from build123d import *

# Parameters (mm, degrees)
SKETCH1_W           = 62
SKETCH1_H           = 42
SKETCH1_W_2         = 41
SKETCH1_H_2         = 21
BOSS_EXTRUDE1_DEPTH = 42
SKETCH2_W           = 4
SKETCH2_H           = 25
BOSS_EXTRUDE2_DEPTH = 4.5
SKETCH2_2_W         = 4
SKETCH2_2_H         = 25
BOSS_EXTRUDE3_DEPTH = 45.55
SKETCH3_W           = 4
SKETCH3_H           = 25
BOSS_EXTRUDE6_DEPTH = 2
SKETCH3_8_W         = 4
SKETCH3_8_H         = 25
BOSS_EXTRUDE7_DEPTH = 53
CUT_EXTRUDE1_DEPTH  = 51
SKETCH_1_W          = 8.5
SKETCH_1_H          = 5.5
CUT_EXTRUDE_1_DEPTH = 40
CUT_EXTRUDE_3_DEPTH = 42
EXTRUDE_1_DEPTH     = 13.5
CUT_EXTRUDE_4_DEPTH = 11.5


with BuildPart() as part:
    # Sketch1 → Boss-Extrude1 (new body)
    with BuildSketch(Plane.XY):
        with Locations((1.904162196, -4.136072895)):
            Rectangle(SKETCH1_W, SKETCH1_H)
        with Locations((1.904162196, -4.136072895)):
            Rectangle(SKETCH1_W_2, SKETCH1_H_2, mode=Mode.SUBTRACT)
    extrude(amount=BOSS_EXTRUDE1_DEPTH)

    # Sketch2 → Boss-Extrude2 (add)
    with BuildSketch(Plane.XY.offset(42)):
        with Locations((-27.095837804, -4.136072895)):
            Rectangle(SKETCH2_W, SKETCH2_H)
    extrude(amount=BOSS_EXTRUDE2_DEPTH)

    # Sketch2_2 → Boss-Extrude3 (add)
    with BuildSketch(Plane.XY.offset(42)):
        with Locations((-27.095837804, -4.136072895)):
            Rectangle(SKETCH2_2_W, SKETCH2_2_H)
    extrude(amount=-BOSS_EXTRUDE3_DEPTH)

    # Sketch3 → Boss-Extrude6 (add)
    with BuildSketch(Plane.XY.offset(46.5)):
        with BuildLine():
            Line((-60.095837804, 4.463927105), (-60.095837804, 8.363927105))
            ThreePointArc((-60.095837804, 8.363927105), (-72.595837804, -4.136072895), (-60.095837804, -16.636072895))
            Line((-60.095837804, -16.636072895), (-60.095837804, -13.176248856))
            Line((-60.095837804, -13.176248856), (-60.555926168, -13.176248856))
            ThreePointArc((-60.555926168, -13.176248856), (-62.055926168, -11.676248856), (-60.555926168, -10.176248856))
            Line((-60.555926168, -10.176248856), (-60.095837804, -10.176248856))
            Line((-60.095837804, -10.176248856), (-60.095837804, -8.186072895))
            ThreePointArc((-60.095837804, -8.186072895), (-64.145837804, -4.136072895), (-60.095837804, -0.086072895))
            Line((-60.095837804, -0.086072895), (-60.095837804, 1.463927105))
            Line((-60.095837804, 1.463927105), (-60.595837804, 1.463927105))
            ThreePointArc((-60.595837804, 1.463927105), (-62.095837804, 2.963927105), (-60.595837804, 4.463927105))
            Line((-60.595837804, 4.463927105), (-60.095837804, 4.463927105))
        make_face()
        with BuildLine():
            ThreePointArc((-68.695837804, -3.636072895), (-67.195837804, -2.136072895), (-65.695837804, -3.636072895))
            Line((-65.695837804, -3.636072895), (-65.695837804, -4.636072895))
            ThreePointArc((-65.695837804, -4.636072895), (-67.195837804, -6.136072895), (-68.695837804, -4.636072895))
            Line((-68.695837804, -4.636072895), (-68.695837804, -3.636072895))
        make_face(mode=Mode.SUBTRACT)
        with BuildLine():
            Line((-29.095837804, -16.636072895), (-29.095837804, 8.363927105))
            Line((-29.095837804, 8.363927105), (-60.095837804, 8.363927105))
            Line((-60.095837804, 8.363927105), (-60.095837804, 4.463927105))
            Line((-60.095837804, 4.463927105), (-59.595837804, 4.463927105))
            ThreePointArc((-59.595837804, 4.463927105), (-58.095837804, 2.963927105), (-59.595837804, 1.463927105))
            Line((-59.595837804, 1.463927105), (-60.095837804, 1.463927105))
            Line((-60.095837804, 1.463927105), (-60.095837804, -0.086072895))
            ThreePointArc((-60.095837804, -0.086072895), (-57.23205534, -1.272290432), (-56.045837804, -4.136072895))
            ThreePointArc((-56.045837804, -4.136072895), (-57.23205534, -6.999855359), (-60.095837804, -8.186072895))
            Line((-60.095837804, -8.186072895), (-60.095837804, -10.176248856))
            Line((-60.095837804, -10.176248856), (-59.635749439, -10.176248856))
            ThreePointArc((-59.635749439, -10.176248856), (-58.135749439, -11.676248856), (-59.635749439, -13.176248856))
            Line((-59.635749439, -13.176248856), (-60.095837804, -13.176248856))
            Line((-60.095837804, -13.176248856), (-60.095837804, -16.636072895))
            Line((-60.095837804, -16.636072895), (-29.095837804, -16.636072895))
        make_face()
        with BuildLine():
            ThreePointArc((-54.495837804, -3.636072895), (-52.995837804, -2.136072895), (-51.495837804, -3.636072895))
            Line((-51.495837804, -3.636072895), (-51.495837804, -4.636072895))
            ThreePointArc((-51.495837804, -4.636072895), (-52.995837804, -6.136072895), (-54.495837804, -4.636072895))
            Line((-54.495837804, -4.636072895), (-54.495837804, -3.636072895))
        make_face(mode=Mode.SUBTRACT)
        with Locations((-27.095837804, -4.136072895)):
            Rectangle(SKETCH3_W, SKETCH3_H)
    extrude(amount=BOSS_EXTRUDE6_DEPTH)

    # Sketch3_8 → Boss-Extrude7 (add)
    with BuildSketch(Plane.XY.offset(46.5)):
        with BuildLine():
            Line((-60.095837804, 4.463927105), (-60.095837804, 8.363927105))
            ThreePointArc((-60.095837804, 8.363927105), (-72.595837804, -4.136072895), (-60.095837804, -16.636072895))
            Line((-60.095837804, -16.636072895), (-60.095837804, -13.176248856))
            Line((-60.095837804, -13.176248856), (-60.555926168, -13.176248856))
            ThreePointArc((-60.555926168, -13.176248856), (-62.055926168, -11.676248856), (-60.555926168, -10.176248856))
            Line((-60.555926168, -10.176248856), (-60.095837804, -10.176248856))
            Line((-60.095837804, -10.176248856), (-60.095837804, -8.186072895))
            ThreePointArc((-60.095837804, -8.186072895), (-64.145837804, -4.136072895), (-60.095837804, -0.086072895))
            Line((-60.095837804, -0.086072895), (-60.095837804, 1.463927105))
            Line((-60.095837804, 1.463927105), (-60.595837804, 1.463927105))
            ThreePointArc((-60.595837804, 1.463927105), (-62.095837804, 2.963927105), (-60.595837804, 4.463927105))
            Line((-60.595837804, 4.463927105), (-60.095837804, 4.463927105))
        make_face()
        with BuildLine():
            ThreePointArc((-68.695837804, -3.636072895), (-67.195837804, -2.136072895), (-65.695837804, -3.636072895))
            Line((-65.695837804, -3.636072895), (-65.695837804, -4.636072895))
            ThreePointArc((-65.695837804, -4.636072895), (-67.195837804, -6.136072895), (-68.695837804, -4.636072895))
            Line((-68.695837804, -4.636072895), (-68.695837804, -3.636072895))
        make_face(mode=Mode.SUBTRACT)
        with BuildLine():
            Line((-29.095837804, -16.636072895), (-29.095837804, 8.363927105))
            Line((-29.095837804, 8.363927105), (-60.095837804, 8.363927105))
            Line((-60.095837804, 8.363927105), (-60.095837804, 4.463927105))
            Line((-60.095837804, 4.463927105), (-59.595837804, 4.463927105))
            ThreePointArc((-59.595837804, 4.463927105), (-58.095837804, 2.963927105), (-59.595837804, 1.463927105))
            Line((-59.595837804, 1.463927105), (-60.095837804, 1.463927105))
            Line((-60.095837804, 1.463927105), (-60.095837804, -0.086072895))
            ThreePointArc((-60.095837804, -0.086072895), (-57.23205534, -1.272290432), (-56.045837804, -4.136072895))
            ThreePointArc((-56.045837804, -4.136072895), (-57.23205534, -6.999855359), (-60.095837804, -8.186072895))
            Line((-60.095837804, -8.186072895), (-60.095837804, -10.176248856))
            Line((-60.095837804, -10.176248856), (-59.635749439, -10.176248856))
            ThreePointArc((-59.635749439, -10.176248856), (-58.135749439, -11.676248856), (-59.635749439, -13.176248856))
            Line((-59.635749439, -13.176248856), (-60.095837804, -13.176248856))
            Line((-60.095837804, -13.176248856), (-60.095837804, -16.636072895))
            Line((-60.095837804, -16.636072895), (-29.095837804, -16.636072895))
        make_face()
        with BuildLine():
            ThreePointArc((-54.495837804, -3.636072895), (-52.995837804, -2.136072895), (-51.495837804, -3.636072895))
            Line((-51.495837804, -3.636072895), (-51.495837804, -4.636072895))
            ThreePointArc((-51.495837804, -4.636072895), (-52.995837804, -6.136072895), (-54.495837804, -4.636072895))
            Line((-54.495837804, -4.636072895), (-54.495837804, -3.636072895))
        make_face(mode=Mode.SUBTRACT)
        with Locations((-27.095837804, -4.136072895)):
            Rectangle(SKETCH3_8_W, SKETCH3_8_H)
    extrude(amount=-BOSS_EXTRUDE7_DEPTH)

    # Sketch3_11 → Cut-Extrude1 (cut)
    with BuildSketch(Plane.XY.offset(46.5)):
        with BuildLine():
            Line((-29.095837804, -16.636072895), (-29.095837804, 8.363927105))
            Line((-29.095837804, 8.363927105), (-60.095837804, 8.363927105))
            Line((-60.095837804, 8.363927105), (-60.095837804, 4.463927105))
            Line((-60.095837804, 4.463927105), (-59.595837804, 4.463927105))
            ThreePointArc((-59.595837804, 4.463927105), (-58.095837804, 2.963927105), (-59.595837804, 1.463927105))
            Line((-59.595837804, 1.463927105), (-60.095837804, 1.463927105))
            Line((-60.095837804, 1.463927105), (-60.095837804, -0.086072895))
            ThreePointArc((-60.095837804, -0.086072895), (-57.23205534, -1.272290432), (-56.045837804, -4.136072895))
            ThreePointArc((-56.045837804, -4.136072895), (-57.23205534, -6.999855359), (-60.095837804, -8.186072895))
            Line((-60.095837804, -8.186072895), (-60.095837804, -10.176248856))
            Line((-60.095837804, -10.176248856), (-59.635749439, -10.176248856))
            ThreePointArc((-59.635749439, -10.176248856), (-58.135749439, -11.676248856), (-59.635749439, -13.176248856))
            Line((-59.635749439, -13.176248856), (-60.095837804, -13.176248856))
            Line((-60.095837804, -13.176248856), (-60.095837804, -16.636072895))
            Line((-60.095837804, -16.636072895), (-29.095837804, -16.636072895))
        make_face()
        with BuildLine():
            ThreePointArc((-54.495837804, -3.636072895), (-52.995837804, -2.136072895), (-51.495837804, -3.636072895))
            Line((-51.495837804, -3.636072895), (-51.495837804, -4.636072895))
            ThreePointArc((-51.495837804, -4.636072895), (-52.995837804, -6.136072895), (-54.495837804, -4.636072895))
            Line((-54.495837804, -4.636072895), (-54.495837804, -3.636072895))
        make_face(mode=Mode.SUBTRACT)
        with BuildLine():
            Line((-60.095837804, 4.463927105), (-60.095837804, 8.363927105))
            ThreePointArc((-60.095837804, 8.363927105), (-72.595837804, -4.136072895), (-60.095837804, -16.636072895))
            Line((-60.095837804, -16.636072895), (-60.095837804, -13.176248856))
            Line((-60.095837804, -13.176248856), (-60.555926168, -13.176248856))
            ThreePointArc((-60.555926168, -13.176248856), (-62.055926168, -11.676248856), (-60.555926168, -10.176248856))
            Line((-60.555926168, -10.176248856), (-60.095837804, -10.176248856))
            Line((-60.095837804, -10.176248856), (-60.095837804, -8.186072895))
            ThreePointArc((-60.095837804, -8.186072895), (-64.145837804, -4.136072895), (-60.095837804, -0.086072895))
            Line((-60.095837804, -0.086072895), (-60.095837804, 1.463927105))
            Line((-60.095837804, 1.463927105), (-60.595837804, 1.463927105))
            ThreePointArc((-60.595837804, 1.463927105), (-62.095837804, 2.963927105), (-60.595837804, 4.463927105))
            Line((-60.595837804, 4.463927105), (-60.095837804, 4.463927105))
        make_face()
        with BuildLine():
            ThreePointArc((-68.695837804, -3.636072895), (-67.195837804, -2.136072895), (-65.695837804, -3.636072895))
            Line((-65.695837804, -3.636072895), (-65.695837804, -4.636072895))
            ThreePointArc((-65.695837804, -4.636072895), (-67.195837804, -6.136072895), (-68.695837804, -4.636072895))
            Line((-68.695837804, -4.636072895), (-68.695837804, -3.636072895))
        make_face(mode=Mode.SUBTRACT)
    extrude(amount=-CUT_EXTRUDE1_DEPTH, mode=Mode.SUBTRACT)

    # Sketch 1 → Cut-Extrude 1 (cut)
    with BuildSketch(Plane(origin=(0, 16.863927105, 0), x_dir=(1, 0, 0), z_dir=(0, 1, 0))):
        with Locations((8.454162196, -32.5)):
            Rectangle(SKETCH_1_W, SKETCH_1_H)
    extrude(amount=-CUT_EXTRUDE_1_DEPTH, mode=Mode.SUBTRACT)

    # Sketch 3 → Cut-Extrude 3 (cut)
    with BuildSketch(Plane(origin=(0, 0, 0), x_dir=(-1, 0, 0), z_dir=(0, 0, -1))):
        Polygon((29.095837804, 8.363927105), (29.095837804, 16.863927105), (-32.904162196, 16.863927105), (-32.904162196, -25.136072895), (29.095837804, -25.136072895), (29.095837804, -16.636072895), (25.095837804, -16.636072895), (25.095837804, 8.363927105), align=None)
    extrude(amount=-CUT_EXTRUDE_3_DEPTH, mode=Mode.SUBTRACT)

    # Sketch 5 → Extrude 1 (add)
    with BuildSketch(Plane(origin=(0, 8.363927105, 0), x_dir=(1, 0, 0), z_dir=(0, 1, 0))):
        Polygon((-25.095837804, 6.5), (-25.095837804, -48.5), (24.904162196, -21), align=None)
    extrude(amount=-EXTRUDE_1_DEPTH)

    # Sketch 5_2 → Cut-Extrude 4 (cut)
    with BuildSketch(Plane(origin=(0, 8.363927105, 0), x_dir=(1, 0, 0), z_dir=(0, 1, 0))):
        Polygon((-25.095837804, 6.5), (-25.095837804, -48.5), (24.904162196, -21), align=None)
    extrude(amount=-CUT_EXTRUDE_4_DEPTH, mode=Mode.SUBTRACT)


solid = part.part
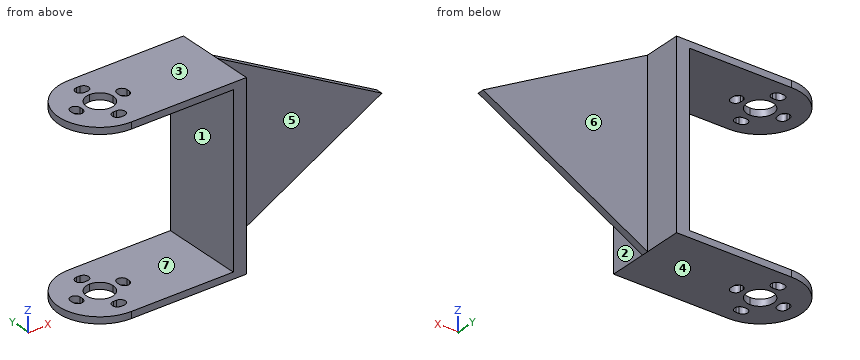
Verification items for the finished model (mm, model axes). Face numbers are marked on the shaded views. A direction names the side the tool comes from. Give positions to 0.01 mm unless a question says otherwise; leave off trailing zeros. Write each loop counter-clockwise with the first axis right and the second up, starting at its lowest first coordinate (ties: lowest second). Pieces come first, ordered by that corner, then holes.
(1) Cross-section at A-A (x = -33.5). Enter the section's corners in (y, z).
(2) Material ranges on line 1 (Z direction, x = -42.5, y = -5); line 2 (X direction, y = -15.25, z = 1); line 3 (Y direction, x = -22, z = 16), recorded low to high.
(3) Gauge pin test, flat ends, axial feed: pin 1 (3.5 mm diameter, centred on y = -11, z = 22.5, fed in from +X); pin 2 (3 mm diameter, centred on x = 6.5, y = -4, fed in from -Z); pin 3 (6 mm diameter, centred on x = -9.5, z = 39.5, fed in from -Y). Record the tip position at first contact, or that the pin passes through.
(4) Cross-section at C-C (z = 18.5). Enter the section's corners in (x, y), plus the area to 3 significant figures.
(5) Cross-section at B-B (y = 3). Enter the section's corners in (x, z).
(6) Access from +Z, -Z, +X, -X, +Y, -Y to the whole of each face (thin tool, end or side, straight path). Record for the marked faces 5, 6 and 7.
(7) Cross-section at D-D (y = -15). Enter the section's corners in (x, z), plus the area to 3 significant figures.
(8) Mould release check, pull along Z, two halves, no side actions. Record for the marked faces 1, 2, 3 and 4: +Z half, -Z half, draft (parallel to the pull), parting line (faces both ways), or undercut.
Worked out:
1. outline: (-16.64, -6.5) - (8.36, -6.5) - (8.36, -4.5) - (-16.64, -4.5) - close; (-16.64, 46.5) - (8.36, 46.5) - (8.36, 48.5) - (-16.64, 48.5) - close
2. line 1: z = -6.5 to -4.5, 46.5 to 48.5
2. line 2: x = -29.1 to -25.1
2. line 3: y = -5.14 to -3.14
3. pin 1: stops at x = -25.1
3. pin 2: stops at z = 10.05
3. pin 3: stops at y = -5.14
4. outline: (-29.1, -16.64) - (-25.1, -16.64) - (-25.1, -5.14) - (20.36, -5.14) - (20.36, -3.14) - (-25.1, -3.14) - (-25.1, 8.36) - (-29.1, 8.36) - close
4. area: 191 mm2
5. outline: (-70.36, -6.5) - (-62.1, -6.5) - (-62.1, -4.5) - (-70.36, -4.5) - close; (-70.36, 46.5) - (-62.1, 46.5) - (-62.1, 48.5) - (-70.36, 48.5) - close; (-58.1, -6.5) - (-25.1, -6.5) - (-25.1, 48.5) - (-58.1, 48.5) - (-58.1, 46.5) - (-29.1, 46.5) - (-29.1, -4.5) - (-58.1, -4.5) - close
6. face 5: +Z, -Z, +X, -Y
6. face 6: +Z, -Z, +X, +Y
6. face 7: -X, +Y, -Y
7. outline: (-66.28, -6.5) - (-25.1, -6.5) - (-25.1, 48.5) - (-66.28, 48.5) - (-66.28, 46.5) - (-29.1, 46.5) - (-29.1, -4.5) - (-66.28, -4.5) - close
7. area: 369 mm2
8. face 1: undercut
8. face 2: draft
8. face 3: +Z half
8. face 4: -Z half
